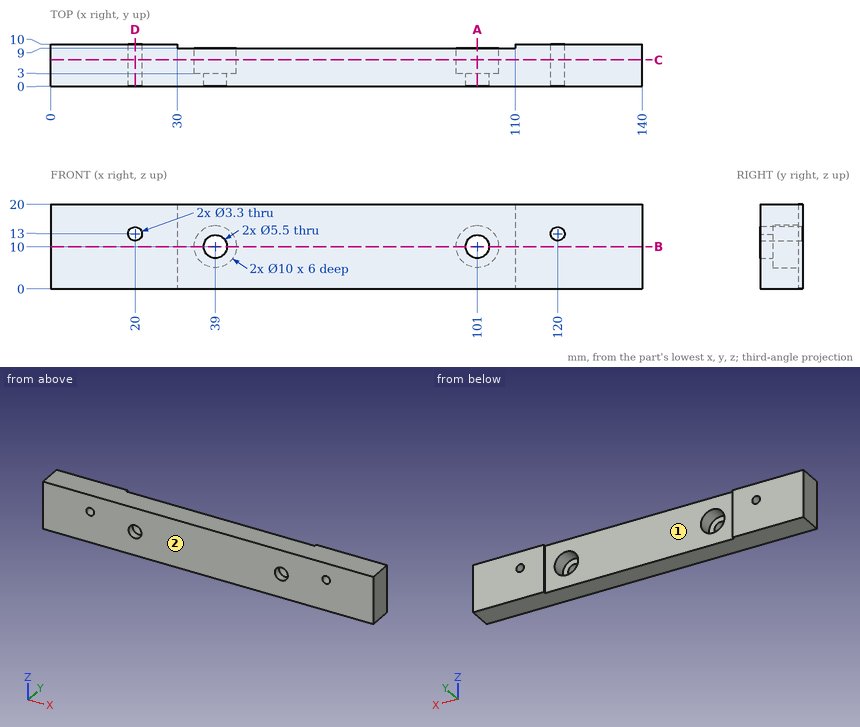
Here's the drawing with two shaded views (mm, measured from the low corner). I have some questions. A direction names the side the tool comes from. Coordinates: 2 decimals unless noted, no trailing zeros. Loops run counter-clockwise (first coordinate to the right, second up) from the corner with the lowest first, then second, coordinate; pieces in that order, holes last. Notation, with made-up numbers: (-2, 16) -> (48, 16) arc R10 cw to (48, 26) -> close; hole circle Ø1 at (48.5, 0.5). An arc over 180 degrees is marked (long way). Use one line per item in the form item = value. Start each with the question number.
(1) On a 3-axis mill with a long thin cutter (end or side, diameter ignored), from which of +Z, -Z, +X, -X, +Y, -Y can I reach the whole of each face in a straight line? I mean the marked faces 1 and 2. Say none if no direction works.
(2) If we section it at B-B (z = 10): Please give me the cut outline in (x, y), then the cut area to 3 significant figures.
(3) If we section it at A-A (x = 101): Please give me the cut outline in (y, z), then the cut area to 4 significant figures.
(4) If we section it at C-C (y = 6.25): Please give me the cut outline in (x, z).
(5) Please list where these lines run through material, in increasing order: line 1 along Z through (x, y) = (20, 2.25); line 2 along X through (y, z) = (4.5, 13); line 3 along X through (y, z) = (4, 7).
(6) If we section it at D-D (x = 20): Please give me the cut outline in (y, z), then the cut area to 3 significant figures.
(7) Will these pins go through, and if not, where does the flat tip stop? pin 1 (12 mm diameter, centred on x = 64.5, z = 5.5, fed in from +Y); pin 2 (9 mm diameter, centred on x = 101, z = 10, fed in from +Y); pin 3 (4.5 mm diameter, centred on x = 39, z = 10, fed in from +Y).
Verdict:
q1.face_1 = +Z, -Z, +Y
q1.face_2 = +Z, -Z, +X, -X, -Y
q2.outline = (0, 0) -> (36.25, 0) -> (36.25, 3) -> (34, 3) -> (34, 9) -> (30, 9) -> (30, 10) -> (0, 10) -> close; (41.75, 0) -> (98.25, 0) -> (98.25, 3) -> (96, 3) -> (96, 9) -> (44, 9) -> (44, 3) -> (41.75, 3) -> close; (103.75, 0) -> (140, 0) -> (140, 10) -> (110, 10) -> (110, 9) -> (106, 9) -> (106, 3) -> (103.75, 3) -> close
q2.area = 1,170 mm²
q3.outline = (0, 0) -> (9, 0) -> (9, 5) -> (3, 5) -> (3, 7.25) -> (0, 7.25) -> close; (0, 12.75) -> (3, 12.75) -> (3, 15) -> (9, 15) -> (9, 20) -> (0, 20) -> close
q3.area = 103.5 mm²
q4.outline = (0, 0) -> (140, 0) -> (140, 20) -> (0, 20) -> close; hole circle Ø3.3 at (20, 13); hole circle Ø10 at (39, 10); hole circle Ø10 at (101, 10); hole circle Ø3.3 at (120, 13)
q5.line_1 = 0 to 11.35, 14.65 to 20
q5.line_2 = 0 to 18.35, 21.65 to 35, 43 to 97, 105 to 118.35, 121.65 to 140
q5.line_3 = 0 to 35, 43 to 97, 105 to 140
q6.outline = (0, 0) -> (10, 0) -> (10, 11.35) -> (0, 11.35) -> close; (0, 14.65) -> (10, 14.65) -> (10, 20) -> (0, 20) -> close
q6.area = 167 mm²
q7.pin_1 = 9
q7.pin_2 = 3
q7.pin_3 = through
